Build history of the part. All positions in model axes, mm. Round coordinates to 2 decimals unless told otherwise and drop trailing zeros. Write each loop counter-clockwise with the first axis right and the second up, starting at its lowest first coordinate (ties: lowest second). Pieces come first, ordered by that corner, then holes. Notation, with made-up numbers: (28.5, 59.5) -> (85.5, 59.5) arc R15 cw to (85.5, 67.5) -> close; hole circle Ø9 at (-20, 44). An arc over 180 degrees is marked (long way). Answer in a Markdown table with one row per item.
```python
from build123d import *

# Parameters (mm, degrees)
BOSS_EXTRUDE1_DEPTH     = 5.75
CUT_EXTRUDE1_DEPTH      = 2.15
CUT_EXTRUDE1_DEPTH_BACK = 11
SKETCH4_R               = 0.25
CHAMFER1_SIZE           = 0.1


with BuildPart() as part:
    # Sketch1 → Boss-Extrude1 (new body, symmetric)
    with BuildSketch(Plane.XY):
        Polygon((-1, 0), (1, 0), (1.15, 1.15), (1, 2.3), (-1, 2.3), (-1.15, 1.15), align=None)
    extrude(amount=BOSS_EXTRUDE1_DEPTH, both=True)

    # Sketch2 → Cut-Extrude1 (cut, two sides)
    with BuildSketch(Plane(origin=(0, 0, 0), x_dir=(0, 0, -1), z_dir=(1, 0, 0))) as cut_extrude1_sk:
        Polygon((5.75, 1.15), (5.6, 2.3), (6.6, 2.3), (6.6, 0), (5.6, 0), align=None)
        Polygon((-5.6, 0), (-5.75, 1.15), (-5.6, 2.3), (-6.6, 2.3), (-6.6, 0), align=None)
    extrude(amount=CUT_EXTRUDE1_DEPTH, mode=Mode.SUBTRACT)
    extrude(cut_extrude1_sk.sketch, amount=-CUT_EXTRUDE1_DEPTH_BACK, mode=Mode.SUBTRACT)

    # Sweep1: sweep along a path in Sketch5
    with BuildLine(Plane(origin=(0, 0, 0), x_dir=(0, 0, -1), z_dir=(1, 0, 0))) as sweep1_path:
        Line((-5, 1.15), (-6.107179677, 1.15))
        ThreePointArc((-6.107179677, 1.15), (-6.257179677, 1.109807621), (-6.366987298, 1))
        Line((-6.366987298, 1), (-6.71339746, 0.4))
        ThreePointArc((-6.71339746, 0.4), (-6.823205081, 0.290192379), (-6.973205081, 0.25))
        Line((-6.973205081, 0.25), (-7.8, 0.25))
    # Sketch4 → Sweep1 (sweep)
    with BuildSketch(Plane.XY.offset(5)):
        with Locations((0, 1.15)):
            Circle(SKETCH4_R)
    sweep1 = sweep(path=sweep1_path.line)

    # Mirror1: Sweep1 across plane
    add(sweep1.mirror(Plane.XY))

    # Chamfer1
    chamfer1_edges = [part.edges().sort_by_distance(p)[0] for p in [
        (-0.25, 0.25, 7.8),
        (-0.25, 0.25, -7.8),
    ]]
    chamfer(chamfer1_edges, length=CHAMFER1_SIZE)


solid = part.part
```
Q1. Two-plate mould, pull along Z, no slides. Class faces 1 (the flat face through (1.074, 0.567, 0.08)), 2 (the flat face through (-0.016, 0.567, -5.674)), 3 (the flat face through (0.016, 1.717, 5.676)): released by +Z, released by -Z, zero draft, split by the parting line, or undercut.
A:
| item | result |
|---|---|
| face 1 | zero draft |
| face 2 | undercut |
| face 3 | released by +Z |
Q2. Wall check: line 1 (Z direction, x = 0.35, y = 1.4); line 2 (X direction, y = 0.55, z = -2); line 3 (Z direction, x = 0.85, y = 2.05). Give the ranges that are in metal, low to high. Write a range as [from, to].
A:
| item | result |
|---|---|
| line 1 | [-5.72, 5.72] |
| line 2 | [-1.07, 1.07] |
| line 3 | [-5.63, 5.63] |
Q3. Saw through at C-C on x = 0.7. Write the cut outline in (y, z).
A:
| item | result |
|---|---|
| outline | (0, -5.6) -> (1.15, -5.75) -> (2.3, -5.6) -> (2.3, 5.6) -> (1.15, 5.75) -> (0, 5.6) -> close |
Q4. Saw through at B-B on z = -0.75. Write the cut outline in (x, y), plus the area to 4 significant figures.
A:
| item | result |
|---|---|
| outline | (-1.15, 1.15) -> (-1, 0) -> (1, 0) -> (1.15, 1.15) -> (1, 2.3) -> (-1, 2.3) -> close |
| area | 4.945 mm² |
Q5. Drop a flat-ended pin along its axis: P1, Ø1, axis at x = 0, y = 1.5, coming from the +Z side. Give the stop position or say it passes through.
A:
| item | result |
|---|---|
| P1 | z = 6.66 |
Q6. Saw through at D-D on y = 2.15. Write the cut outline in (x, z), plus the area to 3 significant figures.
A:
| item | result |
|---|---|
| outline | (-1.02, -5.62) -> (1.02, -5.62) -> (1.02, 5.62) -> (-1.02, 5.62) -> close |
| area | 22.9 mm² |
